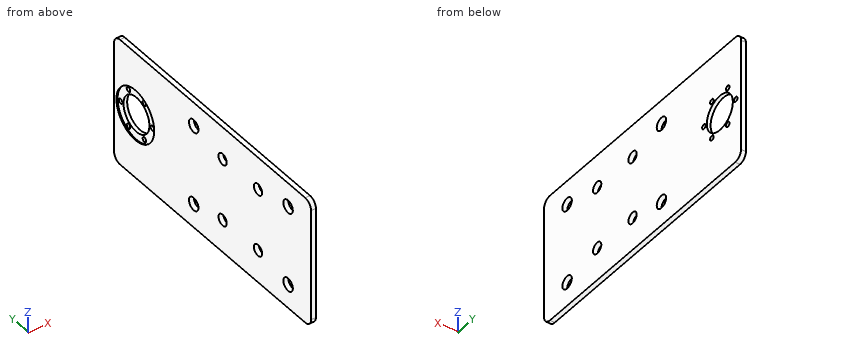
from build123d import *

# Parameters (mm, degrees)
BOSS_EXTRUDE1_DEPTH = 40
SKETCH16_R          = 3.5
SKETCH16_R_2        = 4
CUT_EXTRUDE5_DEPTH  = 150.212253532
SKETCH18_R          = 1.5
SKETCH18_R_2        = 11
CUT_EXTRUDE6_DEPTH  = 150.212253532
SKETCH19_R          = 16
CUT_EXTRUDE7_DEPTH  = 0.7
FILLET1_R           = 5


with BuildPart() as part:
    # Sketch1 → Boss-Extrude1 (new, symmetric)
    with BuildSketch(Plane.XY):
        Polygon((0, -23.280493307), (0, 106.719506693), (0, 143.719506693), (3, 143.719506693), (3, 103.719506693), (3, -23.280493307), align=None)
    extrude(amount=BOSS_EXTRUDE1_DEPTH, both=True)

    # Sketch16 → Cut-Extrude5 (cut, through all)
    with BuildSketch(Plane(origin=(3, 0, 0), x_dir=(0, 0, -1), z_dir=(1, 0, 0))):
        with Locations((-19.5, 21.719506693)):
            Circle(SKETCH16_R)
        with Locations((19.5, 21.719506693)):
            Circle(SKETCH16_R)
        with Locations((19.5, 51.719506693)):
            Circle(SKETCH16_R)
        with Locations((-19.5, 51.719506693)):
            Circle(SKETCH16_R)
        with Locations((25, 76.219506693)):
            Circle(SKETCH16_R_2)
        with Locations((-25, 76.219506693)):
            Circle(SKETCH16_R_2)
        with Locations((-25, -3.780493307)):
            Circle(SKETCH16_R_2)
        with Locations((25, -3.780493307)):
            Circle(SKETCH16_R_2)
    extrude(amount=-CUT_EXTRUDE5_DEPTH, mode=Mode.SUBTRACT)

    # Sketch18 → Cut-Extrude6 (cut, through all)
    with BuildSketch(Plane.ZY):
        with Locations((0, 139.219506693)):
            Circle(SKETCH18_R)
        with Locations((0, 125.719506693)):
            Circle(SKETCH18_R_2)
        with Locations((11.691342951, 132.469506693)):
            Circle(SKETCH18_R)
        with Locations((11.691342951, 118.969506693)):
            Circle(SKETCH18_R)
        with Locations((0, 112.219506693)):
            Circle(SKETCH18_R)
        with Locations((-11.691342951, 118.969506693)):
            Circle(SKETCH18_R)
        with Locations((-11.691342951, 132.469506693)):
            Circle(SKETCH18_R)
    extrude(amount=-CUT_EXTRUDE6_DEPTH, mode=Mode.SUBTRACT)

    # Sketch19 → Cut-Extrude7 (cut)
    with BuildSketch(Plane.ZY):
        with Locations((0, 125.719506693)):
            Circle(SKETCH19_R)
    extrude(amount=-CUT_EXTRUDE7_DEPTH, mode=Mode.SUBTRACT)

    # Fillet1
    fillet1_edges = [part.edges().sort_by_distance(p)[0] for p in [
        (1.5, 143.719506693, 40),
        (1.5, -23.280493307, 40),
        (1.5, 143.719506693, -40),
        (1.5, -23.280493307, -40),
    ]]
    fillet(fillet1_edges, radius=FILLET1_R)


solid = part.part
Source: CAD feature listing. Evaluate the final solid. Frame: model axes, mm. Round coordinates to 2 decimals unless told otherwise and drop trailing zeros. Order: outer loops, then holes, each group sorted by start corner. A loop starts at its lowest first (then second) coordinate and runs counter-clockwise, first axis right, second up. Notation, with made-up numbers: (29, -29.75) - (87, -29.75) arc R24 ccw to (87, 7.25) - close; hole circle Ø9 at (44.5, 23). An arc over 180 degrees is marked (long way). Use a Markdown table: item, result. Add a question column.
1. Section query A-A (z = 0). Return the cut outline in (x, y).
2. First-contact query: pin 1 (4 mm diameter, centred on y = 112.22, z = 0, fed in from +X); pin 2 (4 mm diameter, centred on y = 132.47, z = 11.69, fed in from -X). Flat tips, straight axial feed; report the tip coordinate or a pass-through.
3. Section query C-C (x = 1.75). Give the number of separate pieces and of enclosed holes in the cut face, then the cut area to 3 significant figures.
4. Line query: probe 1 along Y at (x, z) = (2.4, 25); probe 2 along Z at (x, y) = (2.55, 21.5); probe 3 along Y at (x, z) = (1.7, -19.5). Output: solid intervals per line, ascending.
5. Section query B-B (z = 19.5). Return the cut outline in (x, y).
6. Section query D-D (y = 127.5). Return the cut outline in (x, z), then the cut area to 3 significant figures.
Derived:
| question | item | result |
|---|---|---|
| 1 | outline | (0, -23.28) - (3, -23.28) - (3, 110.72) - (0.7, 110.72) - (0.7, 109.72) - (0, 109.72) - close; (0, 141.72) - (0.7, 141.72) - (0.7, 140.72) - (3, 140.72) - (3, 143.72) - (0, 143.72) - close; (0.7, 113.72) - (3, 113.72) - (3, 114.72) - (0.7, 114.72) - close; (0.7, 136.72) - (3, 136.72) - (3, 137.72) - (0.7, 137.72) - close |
| 2 | pin 1 | x = 3 |
| 2 | pin 2 | x = 0.7 |
| 3 | separate pieces | 1 |
| 3 | enclosed holes | 15 |
| 3 | area | 12,600 mm2 |
| 4 | probe 1 | -23.28 to -7.78, 0.22 to 72.22, 80.22 to 143.72 |
| 4 | probe 2 | -40 to -22.99, -16.01 to 16.01, 22.99 to 40 |
| 4 | probe 3 | -23.28 to 18.22, 25.22 to 48.22, 55.22 to 143.72 |
| 5 | outline | (0, -23.28) - (3, -23.28) - (3, 18.22) - (0, 18.22) - close; (0, 25.22) - (3, 25.22) - (3, 48.22) - (0, 48.22) - close; (0, 55.22) - (3, 55.22) - (3, 143.72) - (0, 143.72) - close |
| 6 | outline | (0, -40) - (3, -40) - (3, -10.85) - (0.7, -10.85) - (0.7, -15.9) - (0, -15.9) - close; (0, 15.9) - (0.7, 15.9) - (0.7, 10.85) - (3, 10.85) - (3, 40) - (0, 40) - close |
| 6 | area | 168 mm2 |
